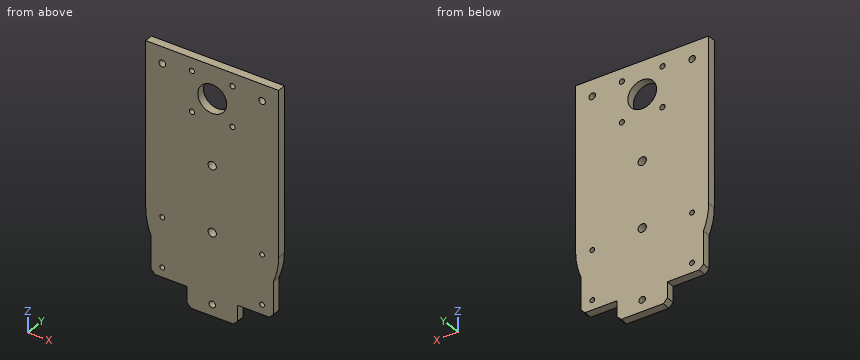
Autodesk Inventor part; units mm, degrees
ref_plane "YZ Plane" through (0, 0, 0) normal (1, 0, 0) x (0, 1, 0)
ref_plane "XZ Plane" through (0, 0, 0) normal (0, 1, 0) x (-1, 0, 0)
ref_plane "XY Plane" through (0, 0, 0) normal (0, 0, 1) x (1, 0, 0)
sketch "Sketch1" plane through (0, 0, 0) normal (0, 1, 0) x (-1, 0, 0)
  line L0 (50.8, -50.8) -> (-50.8, -50.8)
  line L1 (-50.8, -50.8) -> (-50.8, 152.4)
  line L2 (-50.8, 152.4) -> (50.8, 152.4)
  line L3 (50.8, 152.4) -> (50.8, -50.8)
  point P0 (0, 0)
  dimension "d0" = 101.6
  dimension "d1" = 203.2
extrude "Extrusion1" add sketch "Sketch1" along normal blind 6.35
sketch "Sketch2" plane through (0, 6.35, 0) normal (0, 1, 0) x (1, 0, 0)
  line L0 (-50.8, -152.4) -> (50.8, -152.4)
  line L1 (25.4, 0) -> (25.4, -152.4) construction
  circle A0 centre (0, -127) radius 11
  circle A1 centre (0, -76.2) radius 3.175
  circle A2 centre (0, -25.4) radius 3.175
  circle A3 centre (0, -127) radius 11
  line L2 (50.8, -152.4) -> (50.8, 50.8)
  dimension "d4" = 22
  dimension "d5" = 6.35
  dimension "d6" = 50.8
  dimension "d7" = 25.4
  dimension "d10" = 6.35
  dimension "d11" = 50.8
  dimension "d12" = 22
  dimension "d13" = 50.8
  dimension "d14" = 50.8
  dimension "d15" = 50.8
extrude "Extrusion2" cut sketch "Sketch2" against normal through all
sketch "Sketch3" plane through (0, 6.35, 0) normal (0, 1, 0) x (1, 0, 0)
  circle A0 centre (15.5, -111.5) radius 2
  circle A1 centre (15.5, -142.5) radius 2
  circle A2 centre (-15.5, -142.5) radius 2
  circle A3 centre (-15.5, -111.5) radius 2
  point P0 (0, 0)
extrude "Extrusion3" cut sketch "Sketch3" against normal through all
sketch "Sketch4" plane through (0, 0, 0) normal (0, -1, 0) x (1, 0, 0)
  line L0 (50.8, 152.4) -> (-50.8, 152.4)
  line L1 (-50.8, 152.4) -> (-50.8, -50.8)
  circle A0 centre (-38.1, 139.7) radius 2.5146
  circle A1 centre (38.1, 139.7) radius 2.5146
  circle A2 centre (-38.1, -38.1) radius 2.5146
  circle A3 centre (38.1, -38.1) radius 2.5146
  point P0 (0, 0)
  dimension "d18" = 5.0292
  dimension "d19" = 12.7
  dimension "d20" = 12.7
  dimension "d23" = 76.2
  dimension "d26" = 177.8
extrude "Extrusion4" cut sketch "Sketch4" against normal through all
sketch "Sketch5" plane through (0, 6.35, 0) normal (0, 1, 0) x (1, 0, 0)
  circle A0 centre (-38.1, 15.24) radius 1.8542
  circle A1 centre (-38.1, -22.86) radius 1.8542
  circle A2 centre (38.1, 15.24) radius 1.8542
  circle A3 centre (38.1, -22.86) radius 1.8542
  point P0 (0, 0)
extrude "Extrusion5" cut sketch "Sketch5" against normal through all
sketch "Sketch7" plane through (0, 0, 0) normal (0, -1, 0) x (1, 0, 0)
  circle A0 centre (-38.1, -38.1) radius 2.5146
  circle A1 centre (38.1, -38.1) radius 2.5146
  circle A2 centre (0, 76.2) radius 3.175
  circle A3 centre (0, 25.4) radius 3.175
  line L0 (-50.8, -50.8) -> (50.8, -50.8)
  line L1 (50.8, -50.8) -> (50.8, 152.4)
  line L2 (-50.8, 152.4) -> (-50.8, -50.8)
  line L3 (-46.8468, -19.5288) -> (-46.8468, 5.7528)
  line L4 (46.8468, 5.7528) -> (46.8468, -19.5288)
  line L5 (16.1193, -38.1) -> (-16.1193, -38.1)
  line L6 (-19.2943, -34.925) -> (-19.2943, -22.7038)
  line L7 (19.2943, -22.7038) -> (19.2943, -34.925)
  line L8 (43.6718, -22.7038) -> (19.2943, -22.7038)
  line L9 (-19.2943, -22.7038) -> (-43.6718, -22.7038)
  line L10 (19.2943, -34.925) -> (16.1193, -38.1)
  line L11 (-19.2943, -34.925) -> (-16.1193, -38.1)
  line L12 (-43.6718, -22.7038) -> (-46.8468, -19.5288)
  line L13 (46.8468, -19.5288) -> (43.6718, -22.7038)
  arc A4 (-50.8, 25.4) -> (-46.8468, 5.7528) centre (0, 25.4) ccw
  arc A5 (46.8468, 5.7528) -> (50.8, 25.4) centre (0, 25.4) ccw
  arc A6 (3.1734, 76.1008) -> (-3.1734, 76.1008) centre (0, 25.4) ccw
  point P0 (0, 0)
  point P1 (46.8468, -22.7038)
  point P2 (-46.8468, -22.7038)
  point P3 (19.2943, -38.1)
  point P4 (-19.2943, -38.1)
  dimension "d41" = 19.2943
  dimension "d43" = 19.2943
  dimension "d44" = 3.175
  dimension "d45" = 3.175
  dimension "d46" = 3.175
  dimension "d47" = 3.175
  dimension "d48" = 3.175
  dimension "d49" = 3.175
  dimension "d50" = 3.175
  dimension "d51" = 3.175
extrude "Extrusion6" cut sketch "Sketch7" against normal through all contours L2 A4 L3 L12 L9 L6 L11 L5 L10 L7 L8 L13 L4 A5 L1 L0
sketch "Sketch8" plane through (0, 0, 0) normal (0, -1, 0) x (1, 0, 0)
  line L0 (-19.2943, -22.7038) -> (-19.2943, -34.925)
  line L1 (-16.1193, -38.1) -> (16.1193, -38.1)
  line L2 (19.2943, -34.925) -> (19.2943, -22.7038)
  circle A0 centre (0, -29.21) radius 2.5146
  point P0 (0, 0)
  dimension "d54" = 5.0292
  dimension "d55" = 8.89
  dimension "d56" = 19.2943
  dimension "d57" = 19.2943
extrude "Extrusion7" cut sketch "Sketch8" against normal through all
equation "\"d4\" = d12"
equation "\"d14\" = d13"
equation "\"d15\" = d13"
equation "\"d43\" = d41"
equation "\"d56\" = d57"
properties part number "gearBoxBase" material "Polycarbonate, Smoke"
Read the model definition and answer for the solid it produces. Units are mm, in the model's axes. Coordinates: 2 decimals unless noted, no trailing zeros. Write each loop counter-clockwise with the first axis right and the second up, starting at its lowest first coordinate (ties: lowest second). Pieces come first, ordered by that corner, then holes. Notation, with made-up numbers: (30, -5.75) -> (87, -5.75) arc R3 ccw to (87, -1.75) -> close; hole circle Ø2 at (58.25, -7). An arc over 180 degrees is marked (long way). Write item = value, one per line.
(1) Section B-B on y = 3.75 is taken. Count the separate pieces of the cut face and the enclosed holes in it, plus the area to 3 significant figures.
From the geometry:
separate_pieces = 1
enclosed_holes = 14
area = 17,500 mm2
(2) Straight lines are drawn through the part: L1, parallel to X at y = 1.5, z = 139.7; L2, parallel to Z at x = -15.5, y = 2.25; L3, parallel to X at y = 2.25, z = 142.5. For each, find the intervals that lie inside material, in ascending order. Write a range as from..to.
From the geometry:
L1 = -50.8..-40.61, -35.59..35.59, 40.61..50.8
L2 = -38.1..109.5, 113.5..140.5, 144.5..152.4
L3 = -50.8..-17.5, -13.5..13.5, 17.5..50.8
(3) Section C-C on z = 127 is taken. Write down the section's boundary in (x, y), plus the area to 3 significant figures.
From the geometry:
outline = (-50.8, 0) -> (-11, 0) -> (-11, 6.35) -> (-50.8, 6.35) -> close; (11, 0) -> (50.8, 0) -> (50.8, 6.35) -> (11, 6.35) -> close
area = 505 mm2
(4) Section A-A on x = 0 is taken. Write down the section's boundary in (y, z) (3 decimals), plus the area to 3 significant figures.
From the geometry:
outline = (0, -38.1) -> (6.35, -38.1) -> (6.35, -31.725) -> (0, -31.725) -> close; (0, -26.695) -> (6.35, -26.695) -> (6.35, 22.225) -> (0, 22.225) -> close; (0, 28.575) -> (6.35, 28.575) -> (6.35, 73.025) -> (0, 73.025) -> close; (0, 79.375) -> (6.35, 79.375) -> (6.35, 116) -> (0, 116) -> close; (0, 138) -> (6.35, 138) -> (6.35, 152.4) -> (0, 152.4) -> close
area = 957 mm2
(5) Section D-D on z = -15.24 is taken. Write down the section's boundary in (x, y), plus the area to 3 significant figures.
From the geometry:
outline = (-46.85, 0) -> (-39.95, 0) -> (-39.95, 6.35) -> (-46.85, 6.35) -> close; (-36.25, 0) -> (36.25, 0) -> (36.25, 6.35) -> (-36.25, 6.35) -> close; (39.95, 0) -> (46.85, 0) -> (46.85, 6.35) -> (39.95, 6.35) -> close
area = 548 mm2
(6) Given pin 1 Ø4.5 at (x, z) = (38.1, 139.7) entering from -Y; pin 2 Ø1 at (y, z) = (2.5, -2) entering from +X; pin 3 Ø3 at (y, z) = (2, -2) entering from -X; pin 4 Ø1.9 at (y, z) = (4.5, -28) entering from +X, each flat-ended and moving along its own axis, determine where each tip first touches the part or whether it passes through.
From the geometry:
pin_1 = through
pin_2 = 46.85
pin_3 = -46.85
pin_4 = 19.29
